from build123d import *

# Parameters (mm, degrees)
SKETCH1_R      = 1.9558
EXTRUDE1_DEPTH = 12.7
SKETCH2_W      = 0.4953
SKETCH2_H      = 0.8636
FILLET1_R      = 0.254
CHAMFER1_SIZE  = 0.396875


with BuildPart() as part:
    # Sketch1 → Extrude1 (new body, symmetric)
    with BuildSketch(Plane.XY):
        Circle(SKETCH1_R)
    extrude(amount=EXTRUDE1_DEPTH, both=True)

    # Sketch2 → Cut-Revolve1 (revolve, cut)
    with BuildSketch(Plane(origin=(0, 0, 0), x_dir=(1, 0, 0), z_dir=(0, 1, 0))):
        with Locations((1.70815, 11.1252)):
            Rectangle(SKETCH2_W, SKETCH2_H)
    revolve(axis=Axis((0, 0, -10.042474892), (0, 0, 1)), mode=Mode.SUBTRACT)

    # Fillet1
    fillet1_edges = [part.edges().sort_by_distance(p)[0] for p in [
        (-1.9558, 0, -12.7),
    ]]
    fillet(fillet1_edges, radius=FILLET1_R)

    # Chamfer1
    chamfer1_edges = [part.edges().sort_by_distance(p)[0] for p in [
        (-1.9558, 0, 12.7),
    ]]
    chamfer(chamfer1_edges, length=CHAMFER1_SIZE)


solid = part.part
Input: part model. Units: mm. Frame: model coordinates. Coordinates: 2 decimals unless noted, no trailing zeros. Loops run counter-clockwise (first coordinate to the right, second up) from the corner with the lowest first, then second, coordinate; pieces in that order, holes last. Notation, with made-up numbers: (78.25, -3) - (129.25, -3) arc R25 ccw to (129.25, 10) - close; hole circle Ø1 at (9.5, 68). An arc over 180 degrees is marked (long way). Answer in a Markdown table with one row per item. Add a question column.
Item 1: Line query: line 1 along Z through (x, y) = (-1.5, -0.2); line 2 along Y through (x, z) = (1.3, 6); line 3 along Z through (x, y) = (-0.05, 1.75). Output: solid intervals per line, ascending. Write a range as [from, to].
Item 2: Section query A-A on z = -1.25. Return the cut outline in (x, y), then the cut area to 3 significant figures.
Item 3: Mould query, pull axis Z, two halves, no side actions, for faces 1 (the cylindrical face through (1.865, 0.587, 0.966)), 2 (the flat face through (0, 0, 12.7)), 3 (the cylindrical face through (-1.16, -0.89, -11.13)). Classes: released by +Z, released by -Z, zero draft, split by the parting line, or undercut.
Recorded:
| question | item | result |
|---|---|---|
| 1 | line 1 | [-12.7, -11.56], [-10.69, 12.7] |
| 1 | line 2 | [-1.46, 1.46] |
| 1 | line 3 | [-12.7, -11.56], [-10.69, 12.51] |
| 2 | outline | circle Ø3.91 at (0, 0) |
| 2 | area | 12.0 mm^2 |
| 3 | face 1 | zero draft |
| 3 | face 2 | released by +Z |
| 3 | face 3 | undercut |
